```python
from build123d import *

# Parameters (mm, degrees)
PAD006_DEPTH     = 0.2
PRISM003_DEPTH   = 4
PRISM004_DEPTH   = 4
PAD_DEPTH        = 6
HOLE_D           = 3.4
HOLE_DEPTH       = 25
HOLE_CBORE_D     = 5.7
HOLE_CBORE_DEPTH = 3
SKETCH004_R      = 1.25
HOLE001_DEPTH    = 25


with BuildPart() as railnutholes:
    # Sketch009 → Pad006 (new body)
    with BuildSketch(Plane.XY.offset(8)):
        with BuildLine():
            ThreePointArc((1.5, 40), (0, 41.5), (-1.5, 40))
            Line((-1.5, 40), (-1.5, 20))
            ThreePointArc((-1.5, 20), (0, 18.5), (1.5, 20))
            Line((1.5, 20), (1.5, 40))
        make_face()
    extrude(amount=PAD006_DEPTH)

    # Prism003 → Prism003 (join)
    with BuildSketch(Plane(origin=(0, 20, 8), x_dir=(0, 1, 0), z_dir=(0, 0, -1))):
        Polygon((3.35, 0), (1.675, 2.901185), (-1.675, 2.901185), (-3.35, 0), (-1.675, -2.901185), (1.675, -2.901185), align=None)
    extrude(amount=PRISM003_DEPTH)

    # Prism004 → Prism004 (join)
    with BuildSketch(Plane(origin=(0, 40, 8), x_dir=(0, 1, 0), z_dir=(0, 0, -1))):
        Polygon((3.35, 0), (1.675, 2.901185), (-1.675, 2.901185), (-3.35, 0), (-1.675, -2.901185), (1.675, -2.901185), align=None)
    extrude(amount=PRISM004_DEPTH)


with BuildPart() as carriagebasemain:
    # Sketch → Pad (new body)
    with BuildSketch(Plane.XY.offset(6)):
        with BuildLine():
            Line((-16, -7.5), (-16, 7.5))
            ThreePointArc((-13.962963, 9.956759), (-15.424501, 9.095712), (-16, 7.5))
            ThreePointArc((-13.962963, 9.956759), (-7.532196, 13.745367), (-5, 20.766499))
            Line((-5, 20.766499), (-5, 48))
            ThreePointArc((-3, 50), (-4.414214, 49.414214), (-5, 48))
            Line((-3, 50), (3, 50))
            ThreePointArc((5, 48), (4.414214, 49.414214), (3, 50))
            Line((5, 48), (5, 20.766499))
            ThreePointArc((5, 20.766499), (7.532196, 13.745367), (13.962963, 9.956759))
            ThreePointArc((16, 7.5), (15.424501, 9.095712), (13.962963, 9.956759))
            Line((16, 7.5), (16, -7.5))
            ThreePointArc((13.5, -10), (15.267767, -9.267767), (16, -7.5))
            Line((13.5, -10), (-13.5, -10))
            ThreePointArc((-16, -7.5), (-15.267767, -9.267767), (-13.5, -10))
        make_face()
    extrude(amount=-PAD_DEPTH)

    # Sketch → AdditiveLoft section 0
    with BuildSketch(Plane.XY.offset(6)):
        with BuildLine():
            Line((-16, -7.5), (-16, 7.5))
            ThreePointArc((-13.962963, 9.956759), (-15.424501, 9.095712), (-16, 7.5))
            ThreePointArc((-13.962963, 9.956759), (-7.532196, 13.745367), (-5, 20.766499))
            Line((-5, 20.766499), (-5, 48))
            ThreePointArc((-3, 50), (-4.414214, 49.414214), (-5, 48))
            Line((-3, 50), (3, 50))
            ThreePointArc((5, 48), (4.414214, 49.414214), (3, 50))
            Line((5, 48), (5, 20.766499))
            ThreePointArc((5, 20.766499), (7.532196, 13.745367), (13.962963, 9.956759))
            ThreePointArc((16, 7.5), (15.424501, 9.095712), (13.962963, 9.956759))
            Line((16, 7.5), (16, -7.5))
            ThreePointArc((13.5, -10), (15.267767, -9.267767), (16, -7.5))
            Line((13.5, -10), (-13.5, -10))
            ThreePointArc((-16, -7.5), (-15.267767, -9.267767), (-13.5, -10))
        make_face()
    # Sketch001 → AdditiveLoft section 1
    with BuildSketch(Plane.XY.offset(7)):
        with BuildLine():
            Line((-15, -7.5), (-15, 7.5))
            ThreePointArc((-13.68, 8.989161), (-14.622497, 8.494987), (-15, 7.5))
            ThreePointArc((-13.68, 8.989161), (-6.768354, 12.613099), (-4, 19.909674))
            Line((-4, 19.909674), (-4, 48))
            ThreePointArc((-3, 49), (-3.707107, 48.707107), (-4, 48))
            Line((-3, 49), (3, 49))
            ThreePointArc((4, 48), (3.707107, 48.707107), (3, 49))
            Line((4, 48), (4, 19.909674))
            ThreePointArc((4, 19.909674), (6.768354, 12.613099), (13.68, 8.989161))
            ThreePointArc((15, 7.5), (14.622497, 8.494987), (13.68, 8.989161))
            Line((15, 7.5), (15, -7.5))
            ThreePointArc((13.5, -9), (14.56066, -8.56066), (15, -7.5))
            Line((13.5, -9), (-13.5, -9))
            ThreePointArc((-15, -7.5), (-14.56066, -8.56066), (-13.5, -9))
        make_face()
    loft()

    # Hole
    with Locations(Plane.XY.offset(7)):
        with Locations((-5, 7.5), (5, 7.5), (-5, -7.5), (5, -7.5)):
            CounterBoreHole(HOLE_D / 2, HOLE_CBORE_D / 2, HOLE_CBORE_DEPTH, depth=HOLE_DEPTH)

    # Sketch004 → Hole001 (cut)
    with BuildSketch(Plane.XY):
        with Locations((0, 20)):
            Circle(SKETCH004_R)
        with Locations((0, 40)):
            Circle(SKETCH004_R)
    extrude(amount=HOLE001_DEPTH, mode=Mode.SUBTRACT)

    # Boolean: cut RailNutHoles
    add(railnutholes.part, mode=Mode.SUBTRACT)


solid = carriagebasemain.part
```
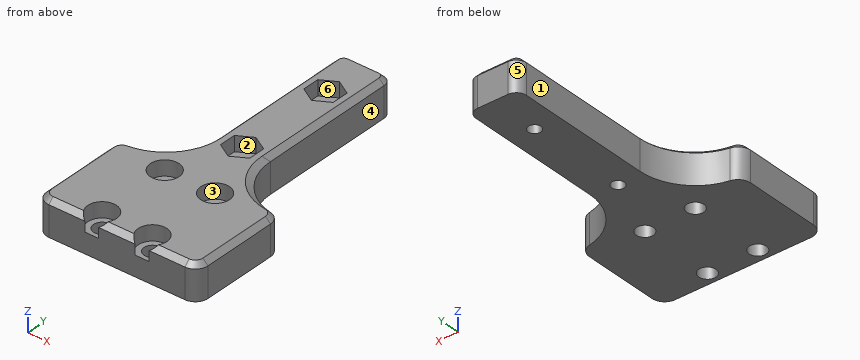
Design review of the part built by this model. Coordinates are the model's own, in mm. Face numbers are marked on the shaded views. A direction names the side the tool comes from. Coordinates: 2 decimals unless noted, no trailing zeros. Answer in a Markdown table with one row per item.
(1) Clearance check with flat-ended pins moving along their axes: pin 1 (1.8 mm diameter, centred on y = 30.5, z = 2, fed in from -X); pin 2 (4.5 mm diameter, centred on x = -5, y = -7.5, fed in from +Z); pin 3 (2.5 mm diameter, centred on y = 20.5, z = 5, fed in from -X); pin 4 (1.5 mm diameter, centred on x = 0, y = 40, fed in from +Z). State where each tip first meets the part, or that it passes through.
Checked values:
| item | result |
|---|---|
| pin 1 | x = -5 |
| pin 2 | z = 4 |
| pin 3 | x = -5.11 |
| pin 4 | through |
(2) The part is to be moulded in two halves that separate along X. For the marked faces 1, 2, 3 and 4, say which applies: released by +X, released by -X, zero draft, split by the parting line, or undercut.
Checked values:
| item | result |
|---|---|
| face 1 | released by -X |
| face 2 | undercut |
| face 3 | undercut |
| face 4 | released by +X |
(3) Wall thickness on line 1 along Y through (x, z) = (-6.5, 3); line 2 along X through (y, z) = (9, 2.25); line 3 along X through (y, z) = (20, 1.6): over which ranges is each line inside the solid? List them lowest first. Write a range as from..to.
Checked values:
| item | result |
|---|---|
| line 1 | -10..-8.3, -6.7..6.7, 8.3..15.22 |
| line 2 | -15.5..-5.8, -4.2..4.2, 5.8..15.5 |
| line 3 | -5.03..-1.25, 1.25..5.03 |
(4) For the marked faces 5 and 6, list the 3-axis set-ups (+Z, -Z, +X, -X, +Y, -Y) from which the entire face can be reached by the end or side of a thin tool; tool diameter is ignored.
Checked values:
| item | result |
|---|---|
| face 5 | +Z, -Z, -X, +Y |
| face 6 | +Z |
